Solid Edge part; units mm, degrees
sketch "Sketch1" plane through (0, 0, 0) normal (0, 0, 1) x (1, 0, 0)
  circle A0 centre (0, 0) radius 6
  circle A1 centre (0, 0) radius 16
extrude "Ajout_matière_1" add sketch "Sketch1" along normal mid plane 10
fillet "Congé_1" radius 1 4 edges at (-16, 0, 5) (-16, 0, -5) (-6, 0, 5) (-6, 0, -5)
properties material "Acier inoxydable"
Source: CAD feature listing. Evaluate the final solid. Frame: model axes, mm. Round coordinates to 2 decimals unless told otherwise and drop trailing zeros. Write each loop counter-clockwise with the first axis right and the second up, starting at its lowest first coordinate (ties: lowest second). Pieces come first, ordered by that corner, then holes. Notation, with made-up numbers: M 80,-29 L 138,-29 A15 ccw 138,-3 Z; hole C 51,-17 d3. An arc over 180 degrees is marked long. Answer as a JSON object with one key per item and string values. Group by question number.
(1) Mould query, pull axis Y, two halves, no side actions, for faces 1 (the cylindrical face through (-6, 0, 0)), 2 (the flat face through (3.1, -6.5, 5)), 3 (the cylindrical face through (-3.47, -15.62, 0.06)). Classes: +Y half, -Y half, draft (parallel to the pull), parting line (faces both ways), or undercut.
(2) Ray query, line 1 (Y direction, x = 0, z = -2); line 2 (Y direction, x = 4, z = -1.5); line 3 (X direction, y = -2, z = 2.5). Return the intervals inside material, ascending. Write a range as [from, to].
(3) Section query A-A on x = 0. Output: boundary loops of the cut face in (y, z).
(4) First-contact query: pin 1 (6 mm diameter, centred on y = 7.5, z = 1, fed in from -X); pin 2 (4 mm diameter, centred on x = -3, z = -1.5, fed in from +Y); pin 3 (2 mm diameter, centred on y = -12.5, z = -2.5, fed in from +X). Flat tips, straight axial feed; report the tip coordinate or a pass-through.
(5) Section query C-C on z = 0. Output: boundary loops of the cut face in (x, y).
Computed values:
{
 "1": {"face 1": "undercut", "face 2": "draft", "face 3": "parting line"},
 "2": {"line 1": "[-16, -6], [6, 16]", "line 2": "[-15.49, -4.47], [4.47, 15.49]", "line 3": "[-15.87, -5.66], [5.66, 15.87]"},
 "3": {"outline": "M -16,-4 A1 ccw -15,-5 L -7,-5 A1 ccw -6,-4 L -6,4 A1 ccw -7,5 L -15,5 A1 ccw -16,4 Z; M 6,-4 A1 ccw 7,-5 L 15,-5 A1 ccw 16,-4 L 16,4 A1 ccw 15,5 L 7,5 A1 ccw 6,4 Z"},
 "4": {"pin 1": "x = -15.35", "pin 2": "y = 15.97", "pin 3": "x = 11.12"},
 "5": {"outline": "C 0,0 d32; hole C 0,0 d12"}
}
